from build123d import *

# Parameters (mm, degrees)
F0_R     = 10
F1_DEPTH = 4
F3_DEPTH = 4
F4_SIZE  = 1


with BuildPart() as f1:
    # F0 (on Top) → F1 (new body)
    with BuildSketch(Plane.XY):
        Circle(F0_R)
    extrude(amount=F1_DEPTH)

    # F2 (on face) → F3 (join)
    with BuildSketch(Plane.XY.offset(4)):
        with BuildLine():
            Line((9.539392, 3), (-9.539392, 3))
            ThreePointArc((-9.539392, 3), (-10, 0), (-9.539392, -3))
            Line((-9.539392, -3), (9.539392, -3))
            ThreePointArc((9.539392, -3), (9.884177, -1.517577), (10, 0))
            ThreePointArc((10, 0), (9.884177, 1.517577), (9.539392, 3))
        make_face()
    extrude(amount=F3_DEPTH)

    # F4
    f4_edges = [f1.edges().sort_by_distance(p)[0] for p in [
        (0, -3, 8),
        (0, 3, 8),
    ]]
    chamfer(f4_edges, length=F4_SIZE)


solid = f1.part
Verification items for the finished model (mm, model axes). A direction names the side the tool comes from. Coordinates: 2 decimals unless noted, no trailing zeros. Order: outer loops, then holes, each group sorted by start corner. A loop starts at its lowest first (then second) coordinate and runs counter-clockwise, first axis right, second up. Notation, with made-up numbers: M 30.5,83 L 78.5,83 A25 ccw 78.5,100 Z; hole C 29,-7.75 d7. An arc over 180 degrees is marked long. One line per item, written item: value. Start each with the question number.
Item 1: Sectioned sample at B-B on z = 4.5. Record the cut outline in (x, y), then the cut area to 3 significant figures.
Item 2: Sectioned sample at D-D on x = -2.25. Record the cut outline in (y, z), then the cut area to 3 significant figures.
Item 3: Sectioned sample at C-C on y = 6. Record the cut outline in (x, z), then the cut area to 3 significant figures.
Item 4: Sectioned sample at A-A on x = 0. Record the cut outline in (y, z), then the cut area to 3 significant figures.
Item 5: Depth check by flat-ended pin: P1, Ø3.5, axis at x = 1, z = 6, coming from the +Y side; P2, Ø3, axis at y = 6, z = 4.5, coming from the -X side; P3, Ø0.9, axis at x = -2, z = 5.5, coming from the -Y side. Enter the tip coordinate at first touch or a pass-through.
Item 6: Access from +Z, -Z, +X, -X, +Y, -Y to the whole of each face (thin tool, end or side, straight path). Record for faces 1 (the flat face through (0, 0, 0)), 2 (the flat face through (0, 3, 5)), 3 (the flat face through (0, -3, 5)).
Item 7: Thickness scan on probe 1 along Y at (x, z) = (2, 1); probe 2 along Y at (x, z) = (-4.5, 6.75); probe 3 along Z at (x, y) = (0.75, -8.5). Record the ranges inside material, lowest first.
Calculated:
1. outline: M -9.54,-3 L 9.54,-3 A10 ccw 10,0 A10 ccw 9.54,3 L -9.54,3 A10 ccw Z
1. area: 118 mm^2
2. outline: M -9.74,0 L 9.74,0 L 9.74,4 L 3,4 L 3,7 L 2,8 L -2,8 L -3,7 L -3,4 L -9.74,4 Z
2. area: 101 mm^2
3. outline: M -8,0 L 8,0 L 8,4 L -8,4 Z
3. area: 64.0 mm^2
4. outline: M -10,0 L 10,0 L 10,4 L 3,4 L 3,7 L 2,8 L -2,8 L -3,7 L -3,4 L -10,4 Z
4. area: 103 mm^2
5. P1: y = 3
5. P2: x = -8.89
5. P3: y = -3
6. face 1: -Z, +X, -X, +Y, -Y
6. face 2: +Z, +X, -X, +Y
6. face 3: +Z, +X, -X, -Y
7. probe 1: -9.8 to 9.8
7. probe 2: -3 to 3
7. probe 3: 0 to 4
